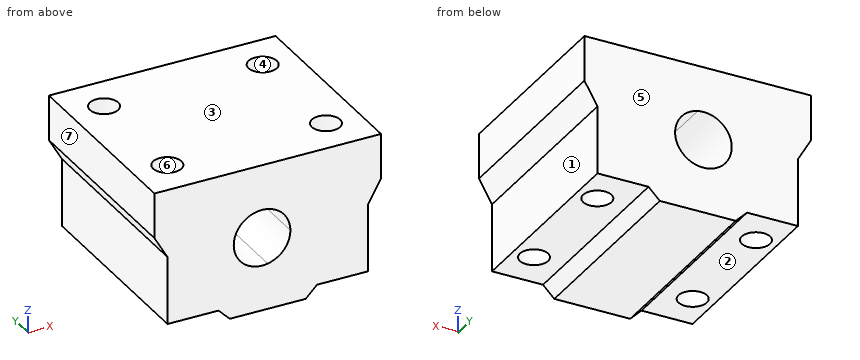
from build123d import *

# Parameters (mm, degrees)
F1_DEPTH = 35
F2_R     = 2.5
F3_DEPTH = 25.4


with BuildPart() as f1:
    # F0 (on Front) → F1 (new body)
    with BuildSketch(Plane.XZ):
        with BuildLine():
            Line((0, -13), (6.690599, -13))
            Line((6.690599, -13), (8.690599, -11))
            Line((8.690599, -11), (17.690599, -11))
            Line((17.690599, -11), (17.690599, 1))
            Line((17.690599, 1), (20, 5))
            Line((20, 5), (20, 13))
            Line((20, 13), (0, 13))
            Line((0, 13), (0, 4.898979))
            ThreePointArc((0, 4.898979), (2.872983, 3.162278), (4, 0))
            ThreePointArc((4, 0), (2.872983, -3.162278), (0, -4.898979))
            Line((0, -4.898979), (0, -13))
        make_face()
        with BuildLine():
            Line((-6.690599, -13), (0, -13))
            Line((0, -13), (0, -4.898979))
            ThreePointArc((0, -4.898979), (-6, 0), (0, 4.898979))
            Line((0, 4.898979), (0, 13))
            Line((0, 13), (-20, 13))
            Line((-20, 13), (-20, 5))
            Line((-20, 5), (-17.690599, 1))
            Line((-17.690599, 1), (-17.690599, -11))
            Line((-17.690599, -11), (-8.690599, -11))
            Line((-8.690599, -11), (-6.690599, -13))
        make_face()
    extrude(amount=F1_DEPTH)

    # F2 (on Top) → F3 (cut, symmetric)
    with BuildSketch(Plane.XY):
        with Locations((14, -28)):
            Circle(F2_R)
        with Locations((14, -7)):
            Circle(F2_R)
        with Locations((-14, -7)):
            Circle(F2_R)
        with Locations((-14, -28)):
            Circle(F2_R)
    extrude(amount=F3_DEPTH, both=True, mode=Mode.SUBTRACT)


solid = f1.part
Can you work these out from the model? Positions are in its coordinate system, mm. Face numbers are marked on the shaded views. A direction names the side the tool comes from. Coordinates: 2 decimals unless noted, no trailing zeros. Write each loop counter-clockwise with the first axis right and the second up, starting at its lowest first coordinate (ties: lowest second). Pieces come first, ordered by that corner, then holes. Notation, with made-up numbers: (78, 36.5) -> (115, 36.5) arc R15 ccw to (115, 54.5) -> close; hole circle Ø3 at (29, -36). An arc over 180 degrees is marked (long way). Write each question's results on one line, items separated by ' | '. Start each with the question number.
Item 1: If we section it at C-C, the plane x = -12: Write out the boundary of the cut face in (y, z), and give its area (3 significant figures).
Item 2: On a 3-axis mill with a long thin cutter (end or side, diameter ignored), from which of +Z, -Z, +X, -X, +Y, -Y can I reach the whole of each face in a straight line? I mean the marked faces 1, 2 and 3. Say none if no direction works.
Item 3: Please list where these lines run through material, in increasing order: probe 1 along Y at (x, z) = (-14, 5.5); probe 2 along Z at (x, y) = (-2, -28); probe 3 along Z at (x, y) = (-1, -27.5).
Item 4: If we section it at A-A, the plane y = -28: Write out the boundary of the cut face in (x, z), and give its area (3 significant figures).
Item 5: Thinking about a two-plate mould opening in Y: for the marked faces 4, 5, 6 and 7, which applies, released by +Y, released by -Y, zero draft, split by the parting line, or undercut?
Item 6: I'm going to push flat-ended pins straight in: P1, Ø2.5, axis at x = -13, y = -21, coming from the -Z side; P2, Ø1, axis at y = -31.5, z = 2.5, coming from the -X side; P3, Ø7, axis at x = 12, y = -18, coming from the -Z side; P4, Ø8, axis at x = 5.5, z = -6.5, coming from the +Y side. Where does each tip first touch, or does it pass through?
Item 7: If we section it at D-D, the plane y = -21.5: Write out the boundary of the cut face in (x, z).
Item 8: If we section it at B-B, the plane x = -1: Write out the boundary of the cut face in (y, z), and give its area (3 significant figures).
Answer block:
1) outline: (-35, -11) -> (-29.5, -11) -> (-29.5, 13) -> (-35, 13) -> close; (-26.5, -11) -> (-8.5, -11) -> (-8.5, 13) -> (-26.5, 13) -> close; (-5.5, -11) -> (0, -11) -> (0, 13) -> (-5.5, 13) -> close | area: 696 mm²
2) face 1: -Z, +X, +Y, -Y | face 2: -Z, -X, +Y, -Y | face 3: +Z, +X, -X, +Y, -Y
3) probe 1: -35 to -30.5, -25.5 to -9.5, -4.5 to 0 | probe 2: -13 to -4.9, 4.9 to 13 | probe 3: -13 to -5, 5 to 13
4) outline: (-20, 5) -> (-17.69, 1) -> (-17.69, -11) -> (-16.5, -11) -> (-16.5, 13) -> (-20, 13) -> close; (-11.5, -11) -> (-8.69, -11) -> (-6.69, -13) -> (6.69, -13) -> (8.69, -11) -> (11.5, -11) -> (11.5, 13) -> (-11.5, 13) -> close; (16.5, -11) -> (17.69, -11) -> (17.69, 1) -> (20, 5) -> (20, 13) -> (16.5, 13) -> close; hole (0, -4.9) arc R5 ccw to (0, 4.9) arc R5 ccw (long way) to start | area: 608 mm²
5) face 4: undercut | face 5: released by +Y | face 6: undercut | face 7: zero draft
6) P1: z = -11 | P2: x = -18.85 | P3: z = -11.19 | P4: y = 0
7) outline: (-20, 5) -> (-17.69, 1) -> (-17.69, -11) -> (-8.69, -11) -> (-6.69, -13) -> (6.69, -13) -> (8.69, -11) -> (17.69, -11) -> (17.69, 1) -> (20, 5) -> (20, 13) -> (-20, 13) -> close; hole (0, -4.9) arc R5 ccw to (0, 4.9) arc R5 ccw (long way) to start
8) outline: (-35, -13) -> (0, -13) -> (0, -5) -> (-35, -5) -> close; (-35, 5) -> (0, 5) -> (0, 13) -> (-35, 13) -> close | area: 560 mm²
